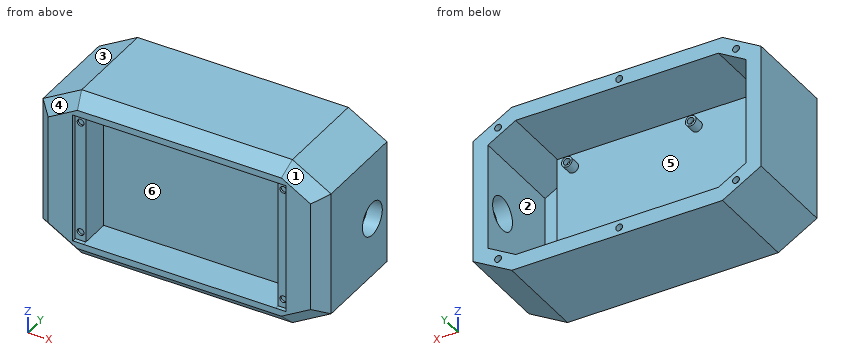
Autodesk Inventor part; units mm, degrees
ref_plane "Work Plane2" through (0, 24, 0) normal (0, 1, 0) x (1, 0, 0)
ref_plane "YZ Plane" through (0, 0, 0) normal (1, 0, 0) x (0, 1, 0)
ref_plane "XZ Plane" through (0, 0, 0) normal (0, 1, 0) x (-1, 0, 0)
sketch "Sketch1" plane through (0, 0, 0) normal (0, 1, 0) x (-1, 0, 0)
  line L0 (0, 0) -> (-95, 0)
  line L1 (-95, 0) -> (-95, -65)
  line L2 (-95, -65) -> (0, -65)
  line L3 (0, -65) -> (0, 0)
  line L4 (0, -65) -> (12.9904, -57.5)
  line L5 (12.9904, -57.5) -> (12.9904, -7.5)
  line L6 (12.9904, -7.5) -> (0, 0)
  line L7 (-95, -65) -> (-107.9904, -57.5)
  line L8 (-107.9904, -57.5) -> (-107.9904, -7.5)
  line L9 (-107.9904, -7.5) -> (-95, 0)
  dimension "d0" = 95
  dimension "d1" = 65
  dimension "d2" = 15
  dimension "d3" = 15
  dimension "d4" = 120
  dimension "d5" = 15
  dimension "d6" = 15
  dimension "d7" = 120
extrude "Extrusion1" add sketch "Sketch1" along normal blind 5
sketch "Sketch2" plane through (0, 5, 0) normal (0, 1, 0) x (1, 0, 0)
  line L0 (1.0001, 63.5) -> (94.0001, 63.5)
  line L1 (94.0001, 63.5) -> (94.0001, 1.5)
  line L2 (94.0001, 1.5) -> (1.0001, 1.5)
  line L3 (1.0001, 1.5) -> (1.0001, 63.5)
  line L4 (0, 0) -> (95, 0)
  line L5 (-12.9904, 57.5) -> (-12.9904, 7.5)
  dimension "d10" = 93
  dimension "d11" = 62
  dimension "d12" = 1.5
  dimension "d13" = 13.9905
extrude "Extrusion2" add sketch "Sketch2" along normal blind 14
sketch "Sketch4" plane through (0, 5, 0) normal (0, 1, 0) x (1, 0, 0)
  line L0 (-12.9904, 57.5) -> (-12.9904, 7.5)
  line L1 (-12.9904, 57.5) -> (-12.9904, 7.5)
  line L2 (-12.9904, 7.5) -> (0, 0)
  line L3 (0, 0) -> (95, 0)
  line L4 (95, 0) -> (107.9904, 7.5)
  line L5 (95, 0) -> (107.9904, 7.5)
  line L6 (107.9904, 7.5) -> (107.9904, 57.5)
  line L7 (107.9904, 57.5) -> (95, 65)
  line L8 (107.9904, 57.5) -> (95, 65)
  line L9 (95, 65) -> (0, 65)
  line L10 (95, 65) -> (0, 65)
  line L11 (0, 65) -> (-12.9904, 57.5)
  line L12 (-19.9904, 61.5415) -> (-19.9904, 3.4585)
  line L13 (114.9904, 61.5415) -> (114.9904, 3.4585)
  line L14 (-1.8756, 72) -> (96.8756, 72)
  line L15 (-19.9904, 61.5415) -> (-1.8756, 72)
  line L16 (96.8756, 72) -> (114.9904, 61.5415)
  line L17 (114.9904, 3.4585) -> (96.8756, -7)
  line L18 (-19.9904, 3.4585) -> (-1.8756, -7)
  line L19 (-1.8756, -7) -> (96.8756, -7)
  line L20 (95, 0) -> (107.9904, 7.5)
  line L21 (107.9904, 7.5) -> (107.9904, 57.5)
  line L22 (0, 0) -> (95, 0)
  dimension "d22" = 7
  dimension "d23" = 7
  dimension "d24" = 7
  dimension "d25" = 7
  dimension "d26" = 7
  dimension "d27" = 7
  dimension "d28" = 7
  dimension "d29" = 7
extrude "Extrusion4" add sketch "Sketch4" along normal blind 45 and the other way blind 5
sketch "Sketch5" plane through (0, 0, 0) normal (0, -1, 0) x (1, 0, 0)
  line L0 (2.4999, -63) -> (92.4999, -63)
  line L1 (92.4999, -63) -> (92.4999, -2)
  line L2 (92.4999, -2) -> (2.4999, -2)
  line L3 (2.4999, -2) -> (2.4999, -63)
  line L4 (0, 0) -> (95, 0)
  line L5 (-12.9904, -57.5) -> (-12.9904, -7.5)
  line L6 (96.8756, 7) -> (-1.8756, 7)
  line L7 (114.9904, -61.5415) -> (114.9904, -3.4585)
  dimension "d34" = 61
  dimension "d35" = 90
  dimension "d43" = 9
  dimension "d44" = 22.4905
extrude "Extrusion5" cut sketch "Sketch5" against normal blind 16
chamfer "Chamfer1" distance 6 angle 45 8 edges at (47.5, 0, -72) (105.933, 0, -66.7707) (114.9904, 0, -32.5) (105.933, 0, 1.7707) (47.5, 0, 7) (-10.933, 0, 1.7707) (-19.9904, 0, -32.5) (-10.933, 0, -66.7707)
sketch "Sketch6" plane through (0, 0, 0) normal (0, -1, 0) x (1, 0, 0)
  line L0 (2.4999, -2) -> (-2.5001, -2)
  line L1 (-2.5001, -2) -> (-2.5001, -63.0139)
  line L2 (-2.5001, -63.0139) -> (2.4999, -63.0139)
  line L3 (2.4999, -63.0139) -> (2.4999, -2)
  line L4 (2.4999, -2) -> (92.4999, -2)
  line L5 (92.4999, -2) -> (97.4999, -2)
  line L6 (97.4999, -2) -> (97.4999, -63.0139)
  line L7 (97.4999, -63.0139) -> (92.4999, -63.0139)
  line L8 (92.4999, -63.0139) -> (92.4999, -2)
  point P0 (0, 0)
  dimension "d45" = 5
  dimension "d46" = 5
extrude "Extrusion6" cut sketch "Sketch6" against normal blind 2
sketch "Sketch7" plane through (0, 2, 0) normal (0, -1, 0) x (1, 0, 0)
  circle A0 centre (-0.0001, -6) radius 1.6
  circle A1 centre (94.9999, -6) radius 1.6
  circle A2 centre (-0.0001, -59.0139) radius 1.6
  circle A3 centre (94.9999, -59.0139) radius 1.6
  line L0 (94.0001, -63.5) -> (94.0001, -1.5)
  line L1 (2.4999, -2) -> (2.4999, -63)
  line L2 (97.4999, -2) -> (97.4999, -63.0139)
  line L3 (-2.5001, -2) -> (97.4999, -2)
  line L4 (-2.5001, -63.0139) -> (-2.5001, -2)
  line L5 (2.4999, -63.0139) -> (-2.5001, -63.0139)
  line L6 (92.4999, -63) -> (92.4999, -2)
  line L7 (97.4999, -63.0139) -> (92.4999, -63.0139)
  point P0 (0, 0)
  dimension "d49" = 3.2
  dimension "d50" = 2.5
  dimension "d51" = 2.5
  dimension "d52" = 4
  dimension "d53" = 0
  dimension "d54" = 2.5
  dimension "d55" = 4
  dimension "d56" = 2.5
  dimension "d57" = 4
extrude "Extrusion7" cut sketch "Sketch7" against normal blind 1 contours A0 | A1 L0 | L0 A1 | L0 A3 | A3 L0 | A2
sketch "Sketch8" plane through (0, 19, 0) normal (0, 1, 0) x (1, 0, 0)
  line L0 (5.0001, 60.5) -> (90.0001, 60.5)
  line L1 (90.0001, 60.5) -> (90.0001, 4.5)
  line L2 (90.0001, 4.5) -> (5.0001, 4.5)
  line L3 (5.0001, 4.5) -> (5.0001, 60.5)
  line L4 (96.8756, 72) -> (-1.8756, 72)
  line L5 (-19.9904, 61.5415) -> (-19.9904, 3.4585)
  circle A0 centre (28.5001, 57) radius 2.5
  circle A1 centre (28.5001, 8) radius 2.5
  circle A2 centre (86.5001, 57) radius 2.5
  circle A3 centre (86.5001, 8) radius 2.5
  circle A4 centre (28.5001, 8) radius 1.6
  circle A5 centre (86.5001, 8) radius 1.6
  circle A6 centre (86.5001, 57) radius 1.6
  circle A7 centre (28.5001, 57) radius 1.6
  circle A8 centre (28.5001, 57) radius 2.5
  point P0 (0, 0)
  dimension "d60" = 85
  dimension "d61" = 56
  dimension "d62" = 11.5
  dimension "d63" = 24.9905
  dimension "d65" = 3.5
  dimension "d66" = 5
  dimension "d68" = 3.5
  dimension "d69" = 3.5
  dimension "d70" = 3.5
  dimension "d71" = 58
  dimension "d72" = 58
  dimension "d75" = 3.5
  dimension "d76" = 3.5
  dimension "d100" = 3.2
  dimension "d101" = 3.2
  dimension "d102" = 3.2
  dimension "d103" = 3.2
extrude "Extrusion8" add sketch "Sketch8" along normal blind 5 contours A0 | A1 | A2 | A3 | A4 | A5 | A6 | A7
sketch "Sketch9" plane through (92.4999, 16, -63) normal (-1, 0, 0) x (0, 0, 1)
  circle A0 centre (49, -5) radius 3.5
  line L0 (61, 0) -> (0, 0)
  line L1 (61, -14) -> (61, 0)
  point P0 (63, -16)
  dimension "d77" = 7
  dimension "d78" = 5
  dimension "d79" = 12
extrude "Extrusion9" cut sketch "Sketch9" against normal blind 5
sketch "Sketch10" plane through (0, 50, 0) normal (0, 1, 0) x (1, 0, 0)
  line L0 (-12.9904, 7.5) -> (-12.9904, 57.5)
  line L1 (-12.9904, 7.5) -> (-16.4904, 1.4378)
  line L2 (-1.8756, -7) -> (-19.9904, 3.4585)
  line L3 (0, 0) -> (95, 0)
  line L4 (0, 0) -> (-3.486, -6.038)
  line L5 (-12.9904, 57.5) -> (0, 65)
  line L6 (-12.9904, 57.5) -> (-16.4904, 63.5622)
  line L7 (-1.8756, 72) -> (-19.9904, 61.5415)
  line L8 (0, 65) -> (-3.5, 71.0622)
  line L9 (0, 65) -> (95, 65)
  line L10 (95, 65) -> (98.5, 71.0622)
  line L11 (114.9904, 61.5415) -> (96.8756, 72)
  line L12 (107.9904, 57.5) -> (95, 65)
  line L13 (107.9904, 57.5) -> (111.4904, 63.5622)
  line L14 (95, 0) -> (107.9904, 7.5)
  line L15 (107.9904, 7.5) -> (111.4904, 1.4378)
  line L16 (95, 0) -> (98.5, -6.0622)
  line L17 (96.8756, -7) -> (114.9904, 3.4585)
  circle A0 centre (103.2452, 0.7189) radius 1.6
  circle A1 centre (103.2452, 64.2811) radius 1.6
  circle A2 centre (-8.2452, 64.2811) radius 1.6
  circle A3 centre (-8.2452, 0.7189) radius 1.6
  circle A4 centre (46.5, -3.5) radius 1.6
  circle A5 centre (46.5, 68.5) radius 1.6
  line L18 (0, 0) -> (-12.9904, 7.5)
  line L19 (-12.9904, 7.5) -> (0, 0)
  line L20 (0, 0) -> (0, -7)
  line L21 (-1.8756, -7) -> (96.8756, -7)
  line L22 (0, 65) -> (0, 72)
  dimension "d82" = 3.2
  dimension "d83" = 7.5
  dimension "d84" = 90
  dimension "d85" = 3.5
  dimension "d86" = 90
  dimension "d87" = 7.5
  dimension "d88" = 3.5
  dimension "d89" = 7.5
  dimension "d90" = 3.5
  dimension "d91" = 7.5
  dimension "d92" = 3.5
  dimension "d93" = 46.5
  dimension "d95" = 46.5
  dimension "d96" = 3.5
  dimension "d97" = 3.5
extrude "Extrusion10" cut sketch "Sketch10" against normal blind 3 contours A0 | A1 | A2 | A3 | A4 | A5
ref_plane "Work Plane2" through (0, 24, 0) normal (0, 1, 0) x (1, 0, 0)
sketch "Sketch14" plane through (0, 24, 0) normal (0, 1, 0) x (1, 0, 0)
  circle A0 centre (28.5001, 8) radius 1.6
  circle A1 centre (28.5001, 8) radius 2.5
  line L0 (28.5001, 8) -> (86.5001, 8)
  line L1 (86.5001, 8) -> (86.5001, 64)
  line L2 (86.5001, 64) -> (28.5001, 64)
  line L3 (28.5001, 64) -> (28.5001, 8)
  point P0 (0, 0)
  dimension "d108" = 3.2
  dimension "d109" = 0
  dimension "d110" = 0
  dimension "d117" = 56
  dimension "d118" = 58
extrude "Extrusion11" cut sketch "Sketch14" against normal blind 2.5 contours L0 L3 A0 | A0 L3 L0
sketch "Sketch15" plane through (86.5001, 24, -8) normal (0, 1, 0) x (1, 0, 0)
  circle A0 centre (0, 0) radius 1.6
  circle A1 centre (0, 49) radius 1.6
  circle A2 centre (0, 49) radius 2.5
  circle A3 centre (-58, 0) radius 1.6
  line L0 (-58, 0) -> (0, 0)
  line L1 (0, 0) -> (0, 49)
  line L2 (0, 49) -> (-58, 49)
  line L3 (-58, 49) -> (-58, 0)
  circle A4 centre (-58, 49) radius 1.6
  point P0 (-86.5001, -8)
  dimension "d113" = 3.2
  dimension "d114" = 3.2
  dimension "d115" = 5
  dimension "d116" = 0
  dimension "d119" = 49
  dimension "d120" = 58
  dimension "d121" = 3.2
extrude "Extrusion12" cut sketch "Sketch15" against normal blind 2.5 contours A0 L0 L1 | L1 L0 A0 | L1 L2 A1 | A1 L2 L1 | A4 L3 L2 | L2 L3 A4
sketch "Sketch16" plane through (107.9904, 5, -57.5) normal (-1, 0, 0) x (0, 0, 1)
  circle A0 centre (23.3152, 33.5) radius 7.8
  line L0 (0, 45) -> (50, 45)
  line L1 (0, 45) -> (50, 45)
  line L2 (57.5, 0) -> (50, 0)
  line L3 (50, 45) -> (50, 0)
  line L4 (50, 0) -> (0, 0)
  line L5 (0, 0) -> (0, 45)
  line L6 (0, 0) -> (0, 45)
  line L7 (-52.9421, -1.2141) -> (6.8536, -5)
  line L8 (6.8536, -5) -> (-57.6878, -5)
  line L9 (-57.6878, -5) -> (10.0174, -1.2141)
  point P0 (57.5, -5)
  dimension "d124" = 15.6
  dimension "d125" = 11.5
extrude "Extrusion13" cut sketch "Sketch16" against normal blind 10 contours A0
properties part number "Bottomv4"
Here's how the part is built. I have some questions about the finished solid (model axes, mm). Face numbers are marked on the shaded views. A direction names the side the tool comes from. Coordinates: 2 decimals unless noted, no trailing zeros. Order: outer loops, then holes, each group sorted by start corner. A loop starts at its lowest first (then second) coordinate and runs counter-clockwise, first axis right, second up.
1) Which directions (+Z, -Z, +X, -X, +Y, -Y) give clear straight access to the entire face, cutting with the end or side of a thin tool? Please do the marked faces 4, 5 and 6.
2) Will these pins go through, and if not, where does the flat tip stop? pin 1 (17.5 mm diameter, centred on x = 53.5, y = 4.5, fed in from +Z); pin 2 (12 mm diameter, centred on x = 5, z = -52.5, fed in from +Y); pin 3 (5.5 mm diameter, centred on x = 29.5, z = -58, fed in from +Y); pin 4 (1.9 mm diameter, centred on x = 28.5, z = -8, fed in from +Y).
3) We'd pull the mould along X, two halves only. Please class the marked faces 1, 2 and 3: +X half, -X half, draft (parallel to the pull), parting line (faces both ways), or undercut.
4) Imagine slicing it at A-A on y = 11. List the corners of the cut face in (x, z) for me, and give its area (3 significant figures).
5) Imagine slicing it at C-C on x = 46.5. List the corners of the cut face in (y, z) for me, and give its area (3 significant figures).
6) Imagine slicing it at B-B on z = -14. List the corners of the cut face in (x, y) for me.
7) Imagine slicing it at D-D on y = 29. List the corners of the cut face in (x, z) for me, and give its area (3 significant figures).
8) I need wall thicknesses on line 1 (Z direction, x = 52, y = 13); line 2 (Z direction, x = 2, y = 6); line 3 (X direction, y = 22, z = -8). Which ranges of each line are inside material? Lowest first, please.
Response values:
1. face 4: +Z, -X, -Y
1. face 5: +Y
1. face 6: -Y
2. pin 1: stops at z = 7
2. pin 2: stops at y = 19
2. pin 3: stops at y = 24
2. pin 4: stops at y = 21.5
3. face 1: +X half
3. face 2: undercut
3. face 3: -X half
4. outline: (-19.99, -61.54) - (-1.88, -72) - (96.88, -72) - (114.99, -61.54) - (114.99, -3.46) - (96.88, 7) - (-1.88, 7) - (-19.99, -3.46) - close; (1, -63.5) - (94, -63.5) - (94, -17.5) - (92.5, -17.5) - (92.5, -63) - (2.5, -63) - (2.5, -2) - (92.5, -2) - (92.5, -10.5) - (94, -10.5) - (94, -1.5) - (1, -1.5) - close; hole (-12.99, -57.5) - (0, -65) - (95, -65) - (107.99, -57.5) - (107.99, -7.5) - (95, 0) - (0, 0) - (-12.99, -7.5) - close
4. area: 2,880 mm2
5. outline: (0, -66) - (6, -72) - (50, -72) - (50, -70.1) - (47, -70.1) - (47, -66.9) - (50, -66.9) - (50, -65) - (5, -65) - (5, -63.5) - (19, -63.5) - (19, -1.5) - (5, -1.5) - (5, 0) - (50, 0) - (50, 1.9) - (47, 1.9) - (47, 5.1) - (50, 5.1) - (50, 7) - (6, 7) - (0, 1) - (0, -2) - (16, -2) - (16, -63) - (0, -63) - close
5. area: 862 mm2
6. outline: (-19.99, 6) - (-13.99, 0) - (-2.5, 0) - (-2.5, 2) - (2.5, 2) - (2.5, 16) - (92.5, 16) - (92.5, 14.5) - (94, 14.5) - (94, 19) - (1, 19) - (1, 5) - (-12.99, 5) - (-12.99, 50) - (-19.99, 50) - close; (92.5, 2) - (97.5, 2) - (97.5, 0) - (108.99, 0) - (114.99, 6) - (114.99, 50) - (107.99, 50) - (107.99, 5) - (94, 5) - (94, 7.5) - (92.5, 7.5) - close
7. outline: (-19.99, -61.54) - (-1.88, -72) - (96.88, -72) - (114.99, -61.54) - (114.99, -3.46) - (96.88, 7) - (-1.88, 7) - (-19.99, -3.46) - close; hole (-12.99, -57.5) - (0, -65) - (95, -65) - (107.99, -57.5) - (107.99, -7.5) - (95, 0) - (0, 0) - (-12.99, -7.5) - close
7. area: 2,620 mm2
8. line 1: z = -72 to -65, -63.5 to -63, -2 to -1.5, 0 to 7
8. line 2: z = -72 to -65, -63.5 to -1.5, 0 to 7
8. line 3: x = -19.99 to -12.99, 26 to 26.9, 30.1 to 31, 84 to 84.9, 88.1 to 89, 107.99 to 114.99
